```python
from build123d import *

# Parameters (mm, degrees)
F1_DEPTH = 82
F2_R     = 9
F3_DEPTH = 25
F4_R     = 30


with BuildPart() as f1:
    # F0 (on Front) → F1 (new body)
    with BuildSketch(Plane.XZ):
        with BuildLine():
            Line((-58.036997, -9.244789), (-58.036997, -15.244789))
            Line((-58.036997, -15.244789), (4.315235, -15.244789))
            ThreePointArc((4.315235, -15.244789), (15.628944, -10.558497), (20.315235, 0.755211))
            Line((20.315235, 0.755211), (20.315235, 37.755211))
            Line((20.315235, 37.755211), (14.315235, 37.755211))
            Line((14.315235, 37.755211), (14.315235, 0.755211))
            ThreePointArc((14.315235, 0.755211), (11.386303, -6.315856), (4.315235, -9.244789))
            Line((4.315235, -9.244789), (-58.036997, -9.244789))
        make_face()
    extrude(amount=F1_DEPTH)

    # F2 (on face) → F3 (cut)
    with BuildSketch(Plane(origin=(0, 0, -15.244789), x_dir=(1, 0, 0), z_dir=(0, 0, -1))):
        with Locations((-23.684765, 26.4)):
            Circle(F2_R)
    extrude(amount=-F3_DEPTH, mode=Mode.SUBTRACT)

    # F4
    f4_edges = [f1.edges().sort_by_distance(p)[0] for p in [
        (-58.036997, 0, -12.244789),
        (17.315235, 0, 37.755211),
    ]]
    fillet(f4_edges, radius=F4_R)


solid = f1.part
```
Geometry: final body of the model. Coordinates: model frame, mm. A direction names the side the tool comes from. Round coordinates to 2 decimals unless told otherwise and drop trailing zeros. Loops run counter-clockwise (first coordinate to the right, second up) from the corner with the lowest first, then second, coordinate; pieces in that order, holes last.
Item 1: Section C-C, the plane y = -55. Output: boundary loops of the cut face in (x, z), plus the area to 3 significant figures.
Checked values:
outline: (-58.04, -15.24) - (4.32, -15.24) arc R16 ccw to (20.32, 0.76) - (20.32, 37.76) - (14.32, 37.76) - (14.32, 0.76) arc R10 cw to (4.32, -9.24) - (-58.04, -9.24) - close
area: 719 mm2
Item 2: Mould query, pull axis Y, two halves, no side actions, for faces 3 (the cylindrical face through (-30.827, -20.924, -12.287)), 4 (the flat face through (17, -56, 37.755)), 5 (the flat face through (-10, -82, -10)), 6 (the cylindrical face through (17.27, -8.55, 28.73)). Classes: released by +Y, released by -Y, zero draft, split by the parting line, or undercut.
Checked values:
face 3: undercut
face 4: zero draft
face 5: released by -Y
face 6: released by +Y
Item 3: Section D-D, the plane z = 4.5. Output: boundary loops of the cut face in (x, y).
Checked values:
outline: (14.32, -82) - (20.32, -82) - (20.32, 0) - (14.32, 0) - close
Item 4: Section B-B, the plane y = -26.4. Output: boundary loops of the cut face in (x, z).
Checked values:
outline: (-57.82, -15.24) - (-32.68, -15.24) - (-32.68, -9.24) - (-57.82, -9.24) - close; (-14.68, -15.24) - (4.32, -15.24) arc R16 ccw to (20.32, 0.76) - (20.32, 37.54) - (14.32, 37.54) - (14.32, 0.76) arc R10 cw to (4.32, -9.24) - (-14.68, -9.24) - close
Item 5: Contact query for flat-ended pins moving along their axis: P1, Ø3, axis at x = -46.5, y = -23, coming from the +Z side; P2, Ø5, axis at x = -23, z = -4.5, coming from the -Y side; P3, Ø4, axis at x = 9, y = -67, coming from the +Z side; P4, Ø5, axis at y = -52, z = -10, coming from the +X side. Output: stop coordinate, or through.
Checked values:
P1: stops at z = -9.24
P2: passes through
P3: stops at z = -6.68
P4: stops at x = 18.02
Item 6: Section A-A, the plane x = -18. Output: boundary loops of the cut face in (y, z), plus the area to 3 significant figures.
Checked values:
outline: (-82, -15.24) - (-33.38, -15.24) - (-33.38, -9.24) - (-82, -9.24) - close; (-19.42, -15.24) - (0, -15.24) - (0, -9.24) - (-19.42, -9.24) - close
area: 408 mm2
Item 7: Line query: L1, parallel to Z at x = -41, y = -70; L2, parallel to X at y = -26.4, z = -10.6; L3, parallel to X at y = -31, z = 5.5. Output: solid intervals per line, ascending.
Checked values:
L1: z = -15.24 to -9.24
L2: x = -57.82 to -32.68, -14.68 to 15.59
L3: x = 14.32 to 20.32
Item 8: Reachability of faces 1 (the flat face through (-27, -40, -15.245)), 2 (the flat face through (-26, -40, -9.245)) from +Z, -Z, +X, -X, +Y, -Y: full face, straight path, thin tool, end or side. Return the list, or none.
Checked values:
face 1: -Z, +X, -X, +Y, -Y
face 2: +Z, -X, +Y, -Y
